Geometry: final body of the model. Coordinates: model frame, mm. A direction names the side the tool comes from. Round coordinates to 2 decimals unless told otherwise and drop trailing zeros. Loops run counter-clockwise (first coordinate to the right, second up) from the corner with the lowest first, then second, coordinate; pieces in that order, holes last. Notation, with made-up numbers: M -33.75,-33.5 L -16.75,-33.5 A34 ccw -16.75,-2.5 Z; hole C 21,-1 d6. An arc over 180 degrees is marked long. Answer as a JSON object with one key per item and string values.
from build123d import *

# Parameters (mm, degrees)
BOSS_EXTRUDE1_DEPTH   = 7
M4X0_7_TAPPED_HOLE1_D = 3.3
SKETCH7_W             = 42
SKETCH7_H             = 14
BOSS_EXTRUDE2_DEPTH   = 20
SKETCH8_R             = 2.5
CUT_EXTRUDE2_DEPTH    = 28


with BuildPart() as part:
    # Sketch1 → Boss-Extrude1 (new, symmetric)
    with BuildSketch(Plane.XY):
        with BuildLine():
            Line((-21, 6.3), (-8.95, 6.3))
            Line((-8.95, 6.3), (-8.95, 33))
            Line((-8.95, 33), (-0.75, 33))
            Line((-0.75, 33), (-0.75, 24.943429983))
            ThreePointArc((-0.75, 24.943429983), (0, 15), (0.75, 24.943429983))
            Line((0.75, 24.943429983), (0.75, 33))
            Line((0.75, 33), (8.95, 33))
            Line((8.95, 33), (8.95, 6.3))
            Line((8.95, 6.3), (21, 6.3))
            Line((21, 6.3), (21, 0))
            Line((21, 0), (-21, 0))
            Line((-21, 0), (-21, 6.3))
        make_face()
    extrude(amount=BOSS_EXTRUDE1_DEPTH, both=True)

    # Sketch4 → CBORE for M4 SHCS2 (revolve, cut)
    with BuildSketch(Plane(origin=(8.95, 28, 0), x_dir=(0, 0, -1), z_dir=(0, 1, 0))):
        Polygon((0, 0), (0, 8.2), (2.25, 8.2), (2.25, 4), (4, 4), (4, 0.25), (4.25, 0), align=None)
    revolve(axis=Axis((15.3, 28, 0), (-1, 0, 0)), mode=Mode.SUBTRACT)

    # M4x0.7 Tapped Hole1 (through all)
    with Locations(Plane(origin=(-0.75, 0, 0), x_dir=(0, 0, -1), z_dir=(1, 0, 0))):
        with Locations((0, 28)):
            Hole(M4X0_7_TAPPED_HOLE1_D / 2)

    # Sketch7 → Boss-Extrude2 (add)
    with BuildSketch(Plane.XZ):
        Rectangle(SKETCH7_W, SKETCH7_H)
    extrude(amount=BOSS_EXTRUDE2_DEPTH)

    # Sketch8 → Cut-Extrude2 (cut)
    with BuildSketch(Plane.XY.offset(7)):
        with Locations((-13, -10)):
            Circle(SKETCH8_R)
        with Locations((13, -10)):
            Circle(SKETCH8_R)
    extrude(amount=-CUT_EXTRUDE2_DEPTH, mode=Mode.SUBTRACT)


solid = part.part
1) Section query B-B (z = 0). Return the cut outline in (x, y), and give its area (3 significant figures).
Results:
{"outline": "M -21,-20 L 21,-20 L 21,6.3 L 8.95,6.3 L 8.95,23.75 L 8.7,24 L 4.95,24 L 4.95,25.75 L 0.75,25.75 L 0.75,24.94 A5 cw long -0.75,24.94 L -0.75,26.35 L -8.95,26.35 L -8.95,6.3 L -21,6.3 Z; M -8.95,29.65 L -0.75,29.65 L -0.75,33 L -8.95,33 Z; M 0.75,30.25 L 4.95,30.25 L 4.95,32 L 8.7,32 L 8.95,32.25 L 8.95,33 L 0.75,33 Z; hole C -13,-10 d5; hole C 13,-10 d5", "area": "1,370 mm2"}
2) Reachability of faces 4 (the flat face through (8.95, 17, 0)), 5 (the cylindrical face through (6.851, 24.034, 0.521)), 6 (the flat face through (-0.75, 30, 0)), 7 (the flat face through (-8.95, 19, 0)) from +Z, -Z, +X, -X, +Y, -Y: full face, straight path, thin tool, end or side. Return the list, or none.
Results:
{"face 4": "+Z, -Z, +X, +Y", "face 5": "+X", "face 6": "+Z, -Z, +Y", "face 7": "+Z, -Z, -X, +Y"}
3) Ray query, line 1 (Y direction, x = 13, z = -3); line 2 (Z direction, x = 7.8, y = 28); line 3 (X direction, y = 20, z = 2). Return the intervals inside material, ascending.
Results:
{"line 1": "-20 to -12.5, -7.5 to 6.3", "line 2": "-7 to -4, 4 to 7", "line 3": "-8.95 to -5, 5 to 8.95"}
4) Section query C-C (y = 28). Return the cut outline in (x, z), and give its area (3 significant figures).
Results:
{"outline": "M -8.95,-7 L -0.75,-7 L -0.75,-1.65 L -8.95,-1.65 Z; M -8.95,1.65 L -0.75,1.65 L -0.75,7 L -8.95,7 Z; M 0.75,-7 L 8.95,-7 L 8.95,-4.25 L 8.7,-4 L 4.95,-4 L 4.95,-2.25 L 0.75,-2.25 Z; M 0.75,2.25 L 4.95,2.25 L 4.95,4 L 8.7,4 L 8.95,4.25 L 8.95,7 L 0.75,7 Z", "area": "152 mm2"}
5) Section query A-A (y = 20). Return the cut outline in (x, z), and give its area (3 significant figures).
Results:
{"outline": "M -8.95,-7 L -5,-7 L -5,7 L -8.95,7 Z; M 5,-7 L 8.95,-7 L 8.95,7 L 5,7 Z", "area": "111 mm2"}
6) Pin query (flat end, axial travel): P1, Ø6, axis at x = 13.5, z = -1, coming from the +Y side; P2, Ø2.5, axis at y = 29, z = 0, coming from the -X side; P3, Ø4, axis at y = 28.5, z = -0.5, coming from the +X side; P4, Ø8, axis at x = -13, y = -10, coming from the +Z side. Return the tip coordinate at first contact, or that it passes through.
Results:
{"P1": "y = 6.3", "P2": "x = -8.95", "P3": "x = 4.95", "P4": "z = 7"}
7) Section query D-D (x = 13). Return the cut outline in (y, z), and give its area (3 significant figures).
Results:
{"outline": "M -20,-7 L -12.5,-7 L -12.5,7 L -20,7 Z; M -7.5,-7 L 6.3,-7 L 6.3,7 L -7.5,7 Z", "area": "298 mm2"}
8) Pull-direction query (X, two-part tool) for faces 1 (the cylindrical face through (0, 15, 0)), 2 (the flat face through (4.95, 30, 2)), 3 (the flat face through (-15, 6.3, 0)); classes: +X half, -X half, draft (parallel to the pull), parting line (faces both ways), or undercut.
Results:
{"face 1": "undercut", "face 2": "+X half", "face 3": "draft"}
